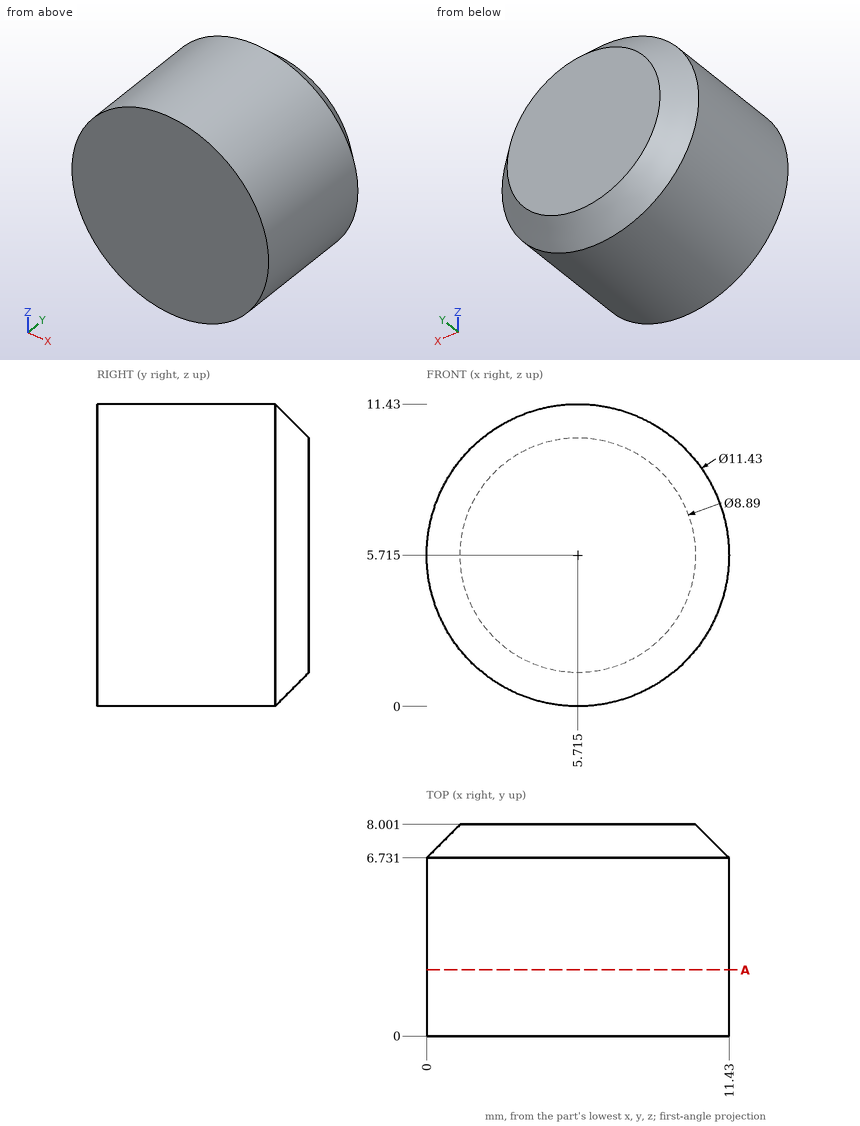
Input: dimensioned drawing with shaded views. Units: mm. Origin: part minimum x, y, z. Give positions to 0.01 mm unless a question says otherwise; leave off trailing zeros. Loops run counter-clockwise (first coordinate to the right, second up) from the corner with the lowest first, then second, coordinate; pieces in that order, holes last. Notation, with made-up numbers: (-27.75, -6.5) -> (-2.75, -6.5) arc R29 ccw to (-2.75, 20.5) -> close; hole circle Ø5 at (74, -10.75). An arc over 180 degrees is marked (long way). Use a Markdown table: item, result. Add a question column.
1) Line query: line 1 along X through (y, z) = (3.5, 9.25); line 2 along X through (y, z) = (2.25, 9); line 3 along Z through (x, y) = (3.75, 0.5). Output: solid intervals per line, ascending. Write a range as [from, to].
2) Section query A-A, the plane y = 2.5. Return the cut outline in (x, z) (3 decimals), then the cut area to 3 significant figures.
3) First-contact query: pin 1 (4 mm diameter, centred on y = 1, z = 6.5, fed in from -X); pin 2 (4 mm diameter, centred on x = 3, y = 3.5, fed in from +Z); pin 3 (2 mm diameter, centred on x = 4.5, y = 2.5, fed in from -Z). Flat tips, straight axial feed; report the tip coordinate or a pass-through.
Numbers:
| question | item | result |
|---|---|---|
| 1 | line 1 | x = [1.22, 10.21] |
| 1 | line 2 | x = [1.04, 10.39] |
| 1 | line 3 | z = [0.35, 11.08] |
| 2 | outline | circle Ø11.43 at (5.715, 5.715) |
| 2 | area | 103 mm2 |
| 3 | pin 1 | stops at x = 0 |
| 3 | pin 2 | stops at z = 11.39 |
| 3 | pin 3 | stops at z = 0 |
